Autodesk Inventor part; units mm, degrees
ref_plane "YZ Plane" through (0, 0, 0) normal (1, 0, 0) x (0, 1, 0)
ref_plane "XZ Plane" through (0, 0, 0) normal (0, 1, 0) x (-1, 0, 0)
ref_plane "XY Plane" through (0, 0, 0) normal (0, 0, 1) x (1, 0, 0)
sketch "Szkic1" plane through (0, 0, 0) normal (0, 1, 0) x (-1, 0, 0)
  line L0 (24.7544, 40.9723) -> (-51.2456, 40.9723)
  line L1 (-51.2456, 40.9723) -> (-51.2456, -15.1007)
  line L2 (-51.2456, -15.1007) -> (24.7544, -15.1007)
  line L3 (24.7544, -15.1007) -> (24.7544, 40.9723)
  point P0 (0, 0)
  dimension "d0" = 76
  dimension "d1" = 56.073
extrude "Wyciągnięcie proste1" add sketch "Szkic1" along normal blind 1.6
fillet "Zaokrąglenie1" radius 1 4 edges at (51.2456, 0.8, -15.1007) (51.2456, 0.8, 40.9723) (-24.7544, 0.8, 40.9723) (-24.7544, 0.8, -15.1007)
sketch "Szkic2" plane through (0, 1.6, 0) normal (0, 1, 0) x (1, 0, 0)
  circle A0 centre (-21.7544, 9.1007) radius 1.6
  circle A1 centre (48.2456, 9.1007) radius 1.6
  circle A2 centre (-21.7544, -37.9723) radius 1.6
  circle A3 centre (48.2456, -37.9723) radius 1.6
  point P0 (0, 0)
hole "Otwór1" at (-21.7544, 1.6, -9.1007) at (48.2456, 1.6, -9.1007) at (-21.7544, 1.6, 37.9723) at (48.2456, 1.6, 37.9723) direction (0, -1, 0) diameter 3 end through all
properties part number "pcb_glowne"
Input: part model. Units: mm. Frame: model coordinates. Round coordinates to 2 decimals unless told otherwise and drop trailing zeros. Answer as CSV lines item,"result". Start each with the question number.
(1) Draft query along Z for faces 1 (the cylindrical face through (46.76, 0.79, -9.3)), 2 (the flat face through (14, 1, -15.101)), 3 (the flat face through (-24.754, 1, 13)). Return one class per face: released by +Z, released by -Z, zero draft, split by the parting line, or undercut.
(2) Line query: line 1 (X direction, y = 0.4, z = 38.5). Output: solid intervals per line, ascending. Write a range as [from, to].
(3) First-contact query: pin 1 (6 mm diameter, centred on x = 8.5, z = 30, fed in from -Y). Flat tip, straight axial feed; report the tip coordinate or a pass-through.
Values found:
1,face 1,"undercut"
1,face 2,"released by -Z"
1,face 3,"zero draft"
2,line 1,"x = [-24.75, -23.16], [-20.35, 46.84], [49.65, 51.25]"
3,pin 1,"stops at y = 0"
